```python
from build123d import *

# Parameters (mm, degrees)
SKETCH1_R            = 4
BOSS_EXTRUDE1_DEPTH  = 2
M4_CLEARANCE_HOLE1_D = 4.5


with BuildPart() as part:
    # Sketch1 → Boss-Extrude1 (new body)
    with BuildSketch(Plane.XY):
        with BuildLine():
            Line((-9.5, 5.5), (9.5, 5.5))
            ThreePointArc((9.5, 5.5), (15, 0), (9.5, -5.5))
            Line((9.5, -5.5), (-9.5, -5.5))
            ThreePointArc((-9.5, -5.5), (-15, 0), (-9.5, 5.5))
        make_face()
        Circle(SKETCH1_R, mode=Mode.SUBTRACT)
    extrude(amount=BOSS_EXTRUDE1_DEPTH)

    # M4 Clearance Hole1 (through all)
    with Locations(Plane.XY.offset(2)):
        with Locations((-9.5, 0), (9.5, 0)):
            Hole(M4_CLEARANCE_HOLE1_D / 2)


solid = part.part
```
Input: part model. Units: mm. Frame: model coordinates. Round coordinates to 2 decimals unless told otherwise and drop trailing zeros. Loops run counter-clockwise (first coordinate to the right, second up) from the corner with the lowest first, then second, coordinate; pieces in that order, holes last.
1) Section query D-D on y = 4.75. Return the cut outline in (x, z).
Ans:
outline: (-12.27, 0) - (12.27, 0) - (12.27, 2) - (-12.27, 2) - close
2) Section query B-B on x = 0. Return the cut outline in (y, z), plus the area to 3 significant figures.
Ans:
outline: (-5.5, 0) - (-4, 0) - (-4, 2) - (-5.5, 2) - close; (4, 0) - (5.5, 0) - (5.5, 2) - (4, 2) - close
area: 6.00 mm2
3) Section query A-A on y = 0. Return the cut outline in (x, z), plus the area to 3 significant figures.
Ans:
outline: (-15, 0) - (-11.75, 0) - (-11.75, 2) - (-15, 2) - close; (-7.25, 0) - (-4, 0) - (-4, 2) - (-7.25, 2) - close; (4, 0) - (7.25, 0) - (7.25, 2) - (4, 2) - close; (11.75, 0) - (15, 0) - (15, 2) - (11.75, 2) - close
area: 26.0 mm2
4) Pull-direction query (X, two-part tool) for faces 1 (the cylindrical face through (-0.867, -3.905, 0.986)), 2 (the cylindrical face through (-15, 0, 1)), 3 (the flat face through (0, 5.5, 1)); classes: released by +X, released by -X, zero draft, split by the parting line, or undercut.
Ans:
face 1: undercut
face 2: released by -X
face 3: zero draft
5) Pin query (flat end, axial travel): pin 1 (2 mm diameter, centred on x = 4.5, y = 2.5, fed in from -Z). Return the tip coordinate at first contact, or that it passes through.
Ans:
pin 1: stops at z = 0
6) Material intervals for line 1 (Y direction, x = 0, z = 1.4); line 2 (X direction, y = 0.5, z = 1.25); line 3 (X direction, y = 0.75, z = 1.5), sorted ascending.
Ans:
line 1: y = -5.5 to -4, 4 to 5.5
line 2: x = -14.98 to -11.69, -7.31 to -3.97, 3.97 to 7.31, 11.69 to 14.98
line 3: x = -14.95 to -11.62, -7.38 to -3.93, 3.93 to 7.38, 11.62 to 14.95
7) Section query C-C on z = 1.5. Return the cut outline in (x, y).
Ans:
outline: (-9.5, -5.5) - (9.5, -5.5) arc R5.5 ccw to (9.5, 5.5) - (-9.5, 5.5) arc R5.5 ccw to start; hole circle Ø4.5 at (-9.5, 0); hole circle Ø8 at (0, 0); hole circle Ø4.5 at (9.5, 0)
